Here's how the part is built. I have some questions about the finished solid (model axes, mm). Face numbers are marked on the shaded views. A direction names the side the tool comes from. Give positions to 0.01 mm unless a question says otherwise; leave off trailing zeros. Order: outer loops, then holes, each group sorted by start corner. A loop starts at its lowest first (then second) coordinate and runs counter-clockwise, first axis right, second up.
from build123d import *

# Parameters (mm, degrees)
BASE_FLANGE1_DEPTH           = 3
SKETCH2_R                    = 8
CUT_EXTRUDE1_DEPTH           = 73.112420355
EDGE_FLANGE1_STRIP_W         = 13.4732
EDGE_FLANGE1_STRIP_H         = 3
EDGE_FLANGE1_STRIP_CUT_DEPTH = 62.933077126
EDGE_FLANGE1_DEPTH           = 62.933077126
EDGE_FLANGE2_STRIP_W         = 13.4732
EDGE_FLANGE2_STRIP_H         = 3
EDGE_FLANGE2_STRIP_CUT_DEPTH = 62.933077126
EDGE_FLANGE2_DEPTH           = 62.933077126
CUT_EXTRUDE14_DEPTH          = 73.492766325
CUT_EXTRUDE15_DEPTH          = 73.492766325
CUT_EXTRUDE16_DEPTH          = 73.492766325
SKETCHED_START               = -2.498589927
SKETCHED_BEND2_DEPTH         = 5
SKETCHED_BEND2_2_DEPTH       = 5


# Read off the part's stored shape, not the designer's step: Sketched Bend2
# Sheet-metal steps are written as plain solids
with BuildPart() as part:
    # Sketch1 → Base-Flange1 (new body)
    with BuildSketch(Plane(origin=(0, 0, 0), x_dir=(1, 0, 0), z_dir=(0, 1, 0))):
        with BuildLine():
            Line((2.501410073, 64.8), (-2.498589927, 64.8))
            Line((-2.498589927, 64.8), (-2.498589927, 44.8))
            Line((-2.498589927, 44.8), (-21.498589927, 44.8))
            ThreePointArc((-21.498589927, 44.8), (-28.847059156, 41.582329983), (-31.466538563, 34))
            Line((-31.466538563, 34), (-31.466538563, -26))
            Line((-31.466538563, -26), (31.466538563, -26))
            Line((31.466538563, -26), (31.466538563, 34))
            ThreePointArc((31.466538563, 34), (28.848015597, 41.581293991), (21.501410073, 44.8))
            Line((21.501410073, 44.8), (2.501410073, 44.8))
            Line((2.501410073, 44.8), (2.501410073, 64.8))
        make_face()
    extrude(amount=-BASE_FLANGE1_DEPTH)

    # Sketch2 → Cut-Extrude1 (cut, through all)
    with BuildSketch(Plane(origin=(0, 0, 0), x_dir=(1, 0, 0), z_dir=(0, 1, 0))):
        with Locations(Location((0.000474376, 21.8, 0), (0, 0, 270))):
            Circle(SKETCH2_R)
    extrude(amount=-CUT_EXTRUDE1_DEPTH, mode=Mode.SUBTRACT)

    # Edge-Flange1 strip (across the edge) → Edge-Flange1 strip cut (cut)
    with BuildSketch(Plane(origin=(-31.466538563, 0, 26), x_dir=(0, 0, -1), z_dir=(1, 0, 0))):
        with Locations((-3, -1.5)):
            Rectangle(EDGE_FLANGE1_STRIP_W, EDGE_FLANGE1_STRIP_H)
    extrude(amount=EDGE_FLANGE1_STRIP_CUT_DEPTH, mode=Mode.SUBTRACT)

    # Edge-Flange1 section (across the edge) → Edge-Flange1 (add)
    with BuildSketch(Plane(origin=(-31.466538563, 0, 26), x_dir=(0, 0, -1), z_dir=(1, 0, 0))):
        with BuildLine():
            Line((0, 0.7366), (0, 2))
            Line((0, 2), (3, 2))
            Line((3, 2), (3, 0.7366))
            ThreePointArc((3, 0.7366), (3.215745145, 0.215745145), (3.7366, 0))
            Line((3.7366, 0), (3.7366, -3))
            ThreePointArc((3.7366, -3), (1.094424801, -1.905575199), (0, 0.7366))
        make_face()
    extrude(amount=EDGE_FLANGE1_DEPTH)

    # Edge-Flange2 strip (across the edge) → Edge-Flange2 strip cut (cut)
    with BuildSketch(Plane(origin=(31.466538563, 2, 26), x_dir=(0, -1, 0), z_dir=(-1, 0, 0))):
        with Locations((-6, -1.5)):
            Rectangle(EDGE_FLANGE2_STRIP_W, EDGE_FLANGE2_STRIP_H)
    extrude(amount=EDGE_FLANGE2_STRIP_CUT_DEPTH, mode=Mode.SUBTRACT)

    # Edge-Flange2 section (across the edge) → Edge-Flange2 (add)
    with BuildSketch(Plane(origin=(31.466538563, 2, 26), x_dir=(0, -1, 0), z_dir=(-1, 0, 0))):
        with BuildLine():
            Line((-3, 0.7366), (-3, 17))
            Line((-3, 17), (0, 17))
            Line((0, 17), (0, 0.7366))
            ThreePointArc((0, 0.7366), (0.215745145, 0.215745145), (0.7366, 0))
            Line((0.7366, 0), (0.7366, -3))
            ThreePointArc((0.7366, -3), (-1.905575199, -1.905575199), (-3, 0.7366))
        make_face()
    extrude(amount=EDGE_FLANGE2_DEPTH)

    # Sketch10 → Cut-Extrude14 (cut, through all)
    with BuildSketch(Plane(origin=(0, 5, 0), x_dir=(1, 0, 0), z_dir=(0, 1, 0))):
        with BuildLine():
            ThreePointArc((-27.999525624, -27.986488127), (-14.471973254, -33.456154948), (0, -35.319999998))
            ThreePointArc((0, -35.319999998), (14.472463109, -33.456275138), (28.000474376, -27.986488127))
            ThreePointArc((28.000474376, -27.986488127), (29.507543106, -29.356635577), (29.415737967, -31.391367011))
            ThreePointArc((29.415737967, -31.391367011), (26.522239798, -32.891637528), (23.552482739, -34.23465141))
            ThreePointArc((23.552482739, -34.23465141), (12.025251123, -37.723725926), (0.039934977, -38.908169509))
            ThreePointArc((0.039934977, -38.908169509), (-11.98559581, -37.731400069), (-23.551533984, -34.234651411))
            ThreePointArc((-23.551533984, -34.234651411), (-26.516212861, -32.894099815), (-29.404911166, -31.396828455))
            ThreePointArc((-29.404911166, -31.396828455), (-29.503369191, -29.361507737), (-27.999525624, -27.986488127))
        make_face()
    extrude(amount=-CUT_EXTRUDE14_DEPTH, mode=Mode.SUBTRACT)

    # Sketch12 → Cut-Extrude15 (cut, through all)
    with BuildSketch(Plane(origin=(0, 5, 0), x_dir=(1, 0, 0), z_dir=(0, 1, 0))):
        with BuildLine():
            add(Edge.make_bspline(
                [(-7.914237019, -39.945550294), (-8.841345223, -39.749796487), (-8.874121397, -38.753829984), (-9.426515507, -38.182603627)],
                knots=[0, 0, 0, 0, 0.911940572, 0.911940572, 0.911940572, 0.911940572], degree=3))
            Line((-7.914237019, -39.945550294), (0, -39.945550294))
            Line((0, -39.945550294), (0, -38.908175729))
            ThreePointArc((0, -38.908175729), (-4.727168745, -38.726119033), (-9.426515507, -38.182603627))
        make_face()
        with BuildLine():
            add(Edge.make_bspline(
                [(-9.426515507, -38.182603627), (-9.479856164, -38.127444478), (-9.538041922, -38.076245756), (-9.602345878, -38.030110388)],
                knots=[0.911940572, 0.911940572, 0.911940572, 0.911940572, 1, 1, 1, 1], degree=3))
            ThreePointArc((-9.426515507, -38.182603627), (-4.727168745, -38.726119033), (0, -38.908175729))
            Line((0, -38.908175729), (0, -38.030110388))
            Line((0, -38.030110388), (-9.602345878, -38.030110388))
        make_face()
        with BuildLine():
            Line((0, -38.030110388), (0, -38.908175729))
            ThreePointArc((0, -38.908175729), (0.019967489, -38.908175848), (0.039934977, -38.908169509))
            ThreePointArc((0.039934977, -38.908169509), (4.746985688, -38.724674098), (9.42633967, -38.182785492))
            add(Edge.make_bspline(
                [(9.42633967, -38.182785492), (9.479728286, -38.127557013), (9.537971255, -38.076296456), (9.602345878, -38.030110388)],
                knots=[0.9118438, 0.9118438, 0.9118438, 0.9118438, 1, 1, 1, 1], degree=3))
            Line((9.602345878, -38.030110388), (0, -38.030110388))
        make_face()
        with BuildLine():
            Line((0, -38.908175729), (0, -39.945550294))
            Line((0, -39.945550294), (7.914237019, -39.945550294))
            add(Edge.make_bspline(
                [(7.914237019, -39.945550294), (8.841246841, -39.74981726), (8.874114431, -38.754041352), (9.42633967, -38.182785492)],
                knots=[0, 0, 0, 0, 0.9118438, 0.9118438, 0.9118438, 0.9118438], degree=3))
            ThreePointArc((9.42633967, -38.182785492), (4.746985688, -38.724674098), (0.039934977, -38.908169509))
            ThreePointArc((0.039934977, -38.908169509), (0.019967489, -38.908175848), (0, -38.908175729))
        make_face()
    extrude(amount=-CUT_EXTRUDE15_DEPTH, mode=Mode.SUBTRACT)

    # Sketch13 → Cut-Extrude16 (cut, through all)
    with BuildSketch(Plane(origin=(0, 5, 0), x_dir=(1, 0, 0), z_dir=(0, 1, 0))):
        with BuildLine():
            Line((-29.503369191, -29.361507737), (-30.236500006, -31.46681125))
            ThreePointArc((-30.236500006, -31.46681125), (-30.1571885, -32.842186741), (-29.128569459, -33.758642374))
            Line((-29.128569459, -33.758642374), (-14.274829355, -38.931167152))
            add(Edge.make_bspline(
                [(-14.274829355, -38.931167152), (-13.356001391, -38.419364556), (-12.413528872, -37.83920993), (-11.311548038, -37.858876708)],
                knots=[0, 0, 0, 0, 1, 1, 1, 1], degree=3))
            Line((-11.311548038, -37.858876708), (-10.639965658, -35.930319464))
            Line((-10.639965658, -35.930319464), (-29.503369191, -29.361507737))
        make_face()
        with BuildLine():
            Line((10.639965658, -35.930319464), (11.311548038, -37.858876708))
            add(Edge.make_bspline(
                [(14.274829355, -38.931167152), (13.356001391, -38.419364556), (12.413528872, -37.83920993), (11.311548038, -37.858876708)],
                knots=[0, 0, 0, 0, 1, 1, 1, 1], degree=3))
            Line((14.274829355, -38.931167152), (29.128569459, -33.758642374))
            ThreePointArc((29.128569459, -33.758642374), (30.1571885, -32.842186741), (30.236500006, -31.46681125))
            Line((30.236500006, -31.46681125), (29.503369191, -29.361507737))
            Line((29.503369191, -29.361507737), (10.639965658, -35.930319464))
        make_face()
    extrude(amount=-CUT_EXTRUDE16_DEPTH, mode=Mode.SUBTRACT)

    # Sketched Bend2 outline → Sketched Bend2 (cut)
    with BuildSketch(Plane.YZ.offset(SKETCHED_START)):
        with BuildLine():
            ThreePointArc((0, -44.8), (-0.845704021, -47.167467001), (-3, -48.463277222))
            Line((-3, -48.463277222), (-3, -64.8))
            Line((-3, -64.8), (0, -64.8))
            Line((0, -64.8), (0, -44.8))
        make_face()
    extrude(amount=SKETCHED_BEND2_DEPTH, mode=Mode.SUBTRACT)

    # Sketched Bend2 2 outline → Sketched Bend2 2 (add)
    with BuildSketch(Plane.YZ.offset(SKETCHED_START)):
        with BuildLine():
            ThreePointArc((-3, -44.8), (-3.215745145, -45.320854855), (-3.7366, -45.5366))
            Line((-3.7366, -45.5366), (-20.223356935, -45.5366))
            Line((-20.223356935, -45.5366), (-20.223356935, -48.5366))
            Line((-20.223356935, -48.5366), (-3.7366, -48.5366))
            ThreePointArc((-3.7366, -48.5366), (-3.36647982, -48.518224121), (-3, -48.463277222))
            Line((-3, -48.463277222), (-3, -44.8))
        make_face()
    extrude(amount=SKETCHED_BEND2_2_DEPTH)


solid = part.part
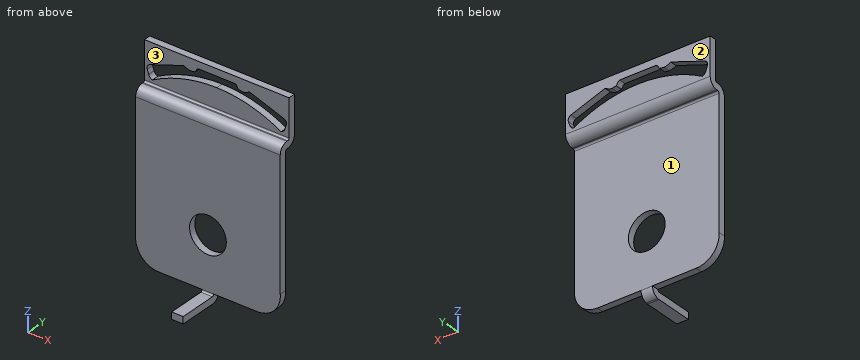
Q1. If we section it at B-B on x = 20: List the corners of the cut face in (y, z) for me.
Filled sheet:
outline: (-3, -44.8) - (0, -44.8) - (0, 22.26) arc R0.74 cw to (0.74, 23) - (1.26, 23) arc R3.74 ccw to (5, 26.74) - (5, 31.7) - (2, 31.7) - (2, 26.74) arc R0.74 cw to (1.26, 26) - (0.74, 26) arc R3.74 ccw to (-3, 22.26) - close; (2, 36.94) - (5, 36.94) - (5, 43) - (2, 43) - close
Q2. For the marked faces 1, 2 and 3, which set-ups out of +Z, -Z, +X, -X, +Y, -Y let a thin tool reach every point of the face, with its end or its side?
Filled sheet:
face 1: -Z, +X, -X, +Y
face 2: +Z, -Z, +X, -X, +Y
face 3: +Z, +X, -X, -Y
Q3. If we section it at C-C on y = -16: List the corners of the cut face in (x, z) for me, plus the area to 3 significant figures.
Filled sheet:
outline: (-2.5, -48.54) - (2.5, -48.54) - (2.5, -45.54) - (-2.5, -45.54) - close
area: 15.0 mm2
Q4. If we section it at D-D on x = -25: List the corners of the cut face in (y, z) for me, plus the area to 3 significant figures.
Filled sheet:
outline: (-3, -44.17) - (0, -44.17) - (0, 22.26) arc R0.74 cw to (0.74, 23) - (1.26, 23) arc R3.74 ccw to (5, 26.74) - (5, 29.56) - (2, 29.56) - (2, 26.74) arc R0.74 cw to (1.26, 26) - (0.74, 26) arc R3.74 ccw to (-3, 22.26) - close; (2, 35.2) - (5, 35.2) - (5, 43) - (2, 43) - close
area: 254 mm2
Q5. If we section it at A-A on z = -21.8: List the corners of the cut face in (x, y) for me.
Filled sheet:
outline: (-31.47, -3) - (-8, -3) - (-8, 0) - (-31.47, 0) - close; (8, -3) - (31.47, -3) - (31.47, 0) - (8, 0) - close
Q6. I'm going to push flat-ended pins straight in: P1, Ø4, axis at x = 0, y = -8.5, coming from the +Z side; P2, Ø3, axis at x = -9, y = 0, coming from the +Z side; P3, Ø19, axis at x = 12, z = -19.5, coming from the +Y side. Where does each tip first touch, or does it pass through?
Filled sheet:
P1: stops at z = -45.54
P2: stops at z = 26.04
P3: stops at y = 0
Q7. I need wall thicknesses on L1, parallel to X at y = -1.95, z = -21.8; L2, parallel to Y at x = 11.5, z = 9; L3, parallel to Z at x = 0.5, y = 1. Which ranges of each line are inside material? Lowest first, please.
Filled sheet:
L1: x = -31.47 to -8, 8 to 31.47
L2: y = -3 to 0
L3: z = 23 to 26
